Can you work these out from the model? Positions are in its coordinate system, mm. A direction names the side the tool comes from. Give positions to 0.01 mm unless a question says otherwise; leave off trailing zeros. Loops run counter-clockwise (first coordinate to the right, second up) from the corner with the lowest first, then second, coordinate; pieces in that order, holes last. Notation, with made-up numbers: (-17.75, 33.25) - (5.25, 33.25) arc R12 cw to (5.25, 52.25) - close; hole circle Ø11 at (59.5, 14). An arc over 180 degrees is marked (long way). Answer as a JSON object with one key per item and string values.
```python
from build123d import *

# Parameters (mm, degrees)
SKETCH_1_W          = 48
SKETCH_1_H          = 20
EXTRUDE_1_DEPTH     = 30
SKETCH_2_W          = 14
SKETCH_2_H          = 30
CUT_EXTRUDE_1_DEPTH = 7
SKETCH_7_W          = 22
SKETCH_7_H          = 30
EXTRUDE_2_DEPTH     = 48
SKETCH_8_W          = 21
SKETCH_8_H          = 30
CUT_EXTRUDE_2_DEPTH = 14
SKETCH_9_W          = 21
SKETCH_9_H          = 30
CUT_EXTRUDE_3_DEPTH = 14
SKETCH_11_W         = 10.4
SKETCH_11_H         = 20.4
CUT_EXTRUDE_4_DEPTH = 56.497747702
SKETCH_13_R         = 4
CUT_EXTRUDE_5_DEPTH = 44.783558558
SKETCH_14_R         = 4
CUT_EXTRUDE_6_DEPTH = 44.783558558
FILLET_1_R          = 7
SKETCH1_W           = 10.4
SKETCH1_H           = 20.4
BOSS_EXTRUDE1_DEPTH = 4
SKETCH_20_R         = 7.5
CUT_EXTRUDE_8_DEPTH = 44.783558558
SKETCH3_R           = 4
CUT_EXTRUDE2_DEPTH  = 57.920997883
CUT_EXTRUDE3_START  = -25
CUT_EXTRUDE3_DEPTH  = 20


with BuildPart() as part:
    # Эскиз1 → Бобышка-Вытянуть1 (new body)
    with BuildSketch(Plane(origin=(0, 0, 0), x_dir=(1, 0, 0), z_dir=(0, 1, 0))):
        Rectangle(SKETCH_1_W, SKETCH_1_H)
    extrude(amount=EXTRUDE_1_DEPTH)

    # Эскиз2 → Вырез-Вытянуть1 (cut)
    with BuildSketch(Plane.XY.offset(10)):
        with Locations((0, 15)):
            Rectangle(SKETCH_2_W, SKETCH_2_H)
    extrude(amount=-CUT_EXTRUDE_1_DEPTH, mode=Mode.SUBTRACT)

    # Эскиз7 → Бобышка-Вытянуть2 (add)
    with BuildSketch(Plane(origin=(24, 0, 0), x_dir=(0, 0, -1), z_dir=(1, 0, 0))):
        with Locations((21, 15)):
            Rectangle(SKETCH_7_W, SKETCH_7_H)
    extrude(amount=-EXTRUDE_2_DEPTH)

    # Эскиз8 → Вырез-Вытянуть2 (cut)
    with BuildSketch(Plane(origin=(24, 0, 0), x_dir=(0, 0, -1), z_dir=(1, 0, 0))):
        with Locations((21.5, 15)):
            Rectangle(SKETCH_8_W, SKETCH_8_H)
    extrude(amount=-CUT_EXTRUDE_2_DEPTH, mode=Mode.SUBTRACT)

    # Эскиз9 → Вырез-Вытянуть3 (cut)
    with BuildSketch(Plane.ZY.offset(24)):
        with Locations((-21.5, 15)):
            Rectangle(SKETCH_9_W, SKETCH_9_H)
    extrude(amount=-CUT_EXTRUDE_3_DEPTH, mode=Mode.SUBTRACT)

    # Эскиз11 → Вырез-Вытянуть4 (cut, through all)
    with BuildSketch(Plane.ZY.offset(10)):
        with Locations((-21.5, 15)):
            Rectangle(SKETCH_11_W, SKETCH_11_H)
    extrude(amount=-CUT_EXTRUDE_4_DEPTH, mode=Mode.SUBTRACT)

    # Эскиз13 → Вырез-Вытянуть5 (cut, through all)
    with BuildSketch(Plane(origin=(0, 0, -11), x_dir=(-1, 0, 0), z_dir=(0, 0, -1))):
        with Locations((17, 15)):
            Circle(SKETCH_13_R)
    extrude(amount=-CUT_EXTRUDE_5_DEPTH, mode=Mode.SUBTRACT)

    # Эскиз14 → Вырез-Вытянуть6 (cut, through all)
    with BuildSketch(Plane(origin=(0, 0, -11), x_dir=(-1, 0, 0), z_dir=(0, 0, -1))):
        with Locations((-17, 15)):
            Circle(SKETCH_14_R)
    extrude(amount=-CUT_EXTRUDE_6_DEPTH, mode=Mode.SUBTRACT)

    # Скругление1
    fillet_1_edges = [part.edges().sort_by_distance(p)[0] for p in [
        (-7, 15, 3),
        (7, 15, 3),
    ]]
    fillet(fillet_1_edges, radius=FILLET_1_R - 0.0001)  # a hair under: the kernel refuses the full size

    # Sketch1 → Boss-Extrude1 (add)
    with BuildSketch(Plane(origin=(10, 0, 0), x_dir=(0, 0, -1), z_dir=(1, 0, 0))):
        with Locations((21.5, 15)):
            Rectangle(SKETCH1_W, SKETCH1_H)
    extrude(amount=-BOSS_EXTRUDE1_DEPTH)

    # Эскиз20 → Вырез-Вытянуть8 (cut, through all)
    with BuildSketch(Plane(origin=(0, 0, -11), x_dir=(-1, 0, 0), z_dir=(0, 0, -1))):
        with Locations((-17, 15)):
            Circle(SKETCH_20_R)
        with Locations((17, 15)):
            Circle(SKETCH_20_R)
    extrude(amount=CUT_EXTRUDE_8_DEPTH, mode=Mode.SUBTRACT)

    # Sketch3 → Cut-Extrude2 (cut, through all)
    with BuildSketch(Plane(origin=(0, 0, -32), x_dir=(-1, 0, 0), z_dir=(0, 0, -1))):
        with Locations(Location((1, 15, 0), (0, 0, 255.522487814))):
            Circle(SKETCH3_R)
    extrude(amount=-CUT_EXTRUDE2_DEPTH, mode=Mode.SUBTRACT)

    # Sketch4 → Cut-Extrude3 (cut)
    with BuildSketch(Plane(origin=(0, 0, -32), x_dir=(-1, 0, 0), z_dir=(0, 0, -1)).offset(CUT_EXTRUDE3_START)):
        Polygon((1, 22.35), (-5.365286718, 18.675), (-5.365286718, 11.325), (1, 7.65), (7.365286718, 11.325), (7.365286718, 18.675), align=None)
    extrude(amount=-CUT_EXTRUDE3_DEPTH, mode=Mode.SUBTRACT)


solid = part.part
```
1) I need wall thicknesses on L1, parallel to Y at x = 17, z = -2; L2, parallel to Z at x = -2, y = 21; L3, parallel to X at y = 15, z = -14. Which ranges of each line are inside material? Lowest first, please.
Check sheet entries:
{"L1": "0 to 11, 19 to 30", "L2": "-32 to -26.7, -16.3 to -7", "L3": "-9.5 to -5, 3 to 9.5"}
2) If we mould it in two halves opening along Y, with no side actions, what happens to faces 5 (the flat face through (-24, 15, 0)), 6 (the flat face through (0, 0, -6)), 7 (the cylindrical face through (-1, 11, -12))? For each: released by +Y, released by -Y, zero draft, split by the parting line, or undercut.
Check sheet entries:
{"face 5": "zero draft", "face 6": "released by -Y", "face 7": "undercut"}
3) Imagine slicing it at B-B on z = 2. Write out the boundary of the cut face in (x, y) (3 decimals), and give its area (3 significant figures).
Check sheet entries:
{"outline": "(-24, 0) - (24, 0) - (24, 30) - (-24, 30) - close; hole circle Ø8 at (-17, 15); hole (-7.365, 11.325) - (-1, 7.65) - (5.365, 11.325) - (5.365, 18.675) - (-1, 22.35) - (-7.365, 18.675) - close; hole circle Ø8 at (17, 15)", "area": "1,200 mm2"}
4) Imagine slicing it at A-A on y = 15. Give the number of separate pieces and of enclosed holes in the cut face, and give its area (3 significant figures).
Check sheet entries:
{"separate pieces": "5", "enclosed holes": "0", "area": "572 mm2"}
5) Imagine slicing it at C-C on x = -17. Write out the boundary of the cut face in (y, z).
Check sheet entries:
{"outline": "(0, -11) - (11, -11) - (11, 10) - (0, 10) - close; (19, -11) - (30, -11) - (30, 10) - (19, 10) - close"}
6) Imagine slicing it at D-D on x = -8.5. Write out the boundary of the cut face in (y, z).
Check sheet entries:
{"outline": "(0, -32) - (30, -32) - (30, 10) - (0, 10) - close; hole (4.8, -26.7) - (25.2, -26.7) - (25.2, -16.3) - (4.8, -16.3) - close"}
7) Which directions (+Z, -Z, +X, -X, +Y, -Y) give clear straight access to the entire face, cutting with the end or side of a thin tool? Please do faces 1 (the cylindrical face through (-5, 24.5, 5.1)), 2 (the flat face through (-4.138, 9.462, -0.508)), 3 (the flat face through (6, 15, -21)), 4 (the cylindrical face through (-9.5, 15, -13.6)).
Check sheet entries:
{"face 1": "+Z, +Y, -Y", "face 2": "+Z", "face 3": "-X", "face 4": "-Z, -X"}
8) I'm going to push flat-ended pins straight in: P1, Ø6, axis at y = 7, z = -23, coming from the +X side; P2, Ø13, axis at x = 17, y = 15, coming from the -Z side; P3, Ø4, axis at y = 4, z = -26, coming from the -X side. Where does each tip first touch, or does it pass through?
Check sheet entries:
{"P1": "x = 10", "P2": "z = -11", "P3": "x = -10"}
